Geometry check sheet. Reference: drawing and pictorial views, mm from the part's lowest x, y, z. A direction names the side the tool comes from. Give positions to 0.01 mm unless a question says otherwise; leave off trailing zeros. Write each loop counter-clockwise with the first axis right and the second up, starting at its lowest first coordinate (ties: lowest second). Pieces come first, ordered by that corner, then holes. Notation, with made-up numbers: M 14.5,-2.5 L 71.5,-2.5 A14 ccw 71.5,22.5 Z; hole C 50,51.5 d10. An arc over 180 degrees is marked long. Write item = value, one per line. Start each with the question number.
1) Cross-section at D-D, the plane x = 31. Record the cut outline in (y, z).
2) Cross-section at C-C, the plane z = 6. Record the cut outline in (x, y), plus the area to 3 significant figures.
3) Go/stop test with flat-tipped pins: pin 1 (1.5 mm diameter, centred on x = 13.5, y = 30.5, fed in from -Z); pin 2 (5 mm diameter, centred on x = 9.5, z = 20.5, fed in from +Y); pin 3 (12 mm diameter, centred on x = 8.5, y = 18.5, fed in from -Z); pin 4 (0.9 mm diameter, centred on x = 5.5, y = 36.5, fed in from -Z). Record where each tip stops, or that it passes through.
4) Access from +Z, -Z, +X, -X, +Y, -Y to the whole of each face (thin tool, end or side, straight path). Record for the marked faces 1 and 2.
5) Scan lines: line 1 along Y through (x, z) = (5.5, 24.4); line 2 along Y through (x, z) = (36, 24). Record each from-to range of solid material in increasing order. Write a range as [from, to].
6) Cross-section at A-A, the plane x = 21. Record the cut outline in (y, z).
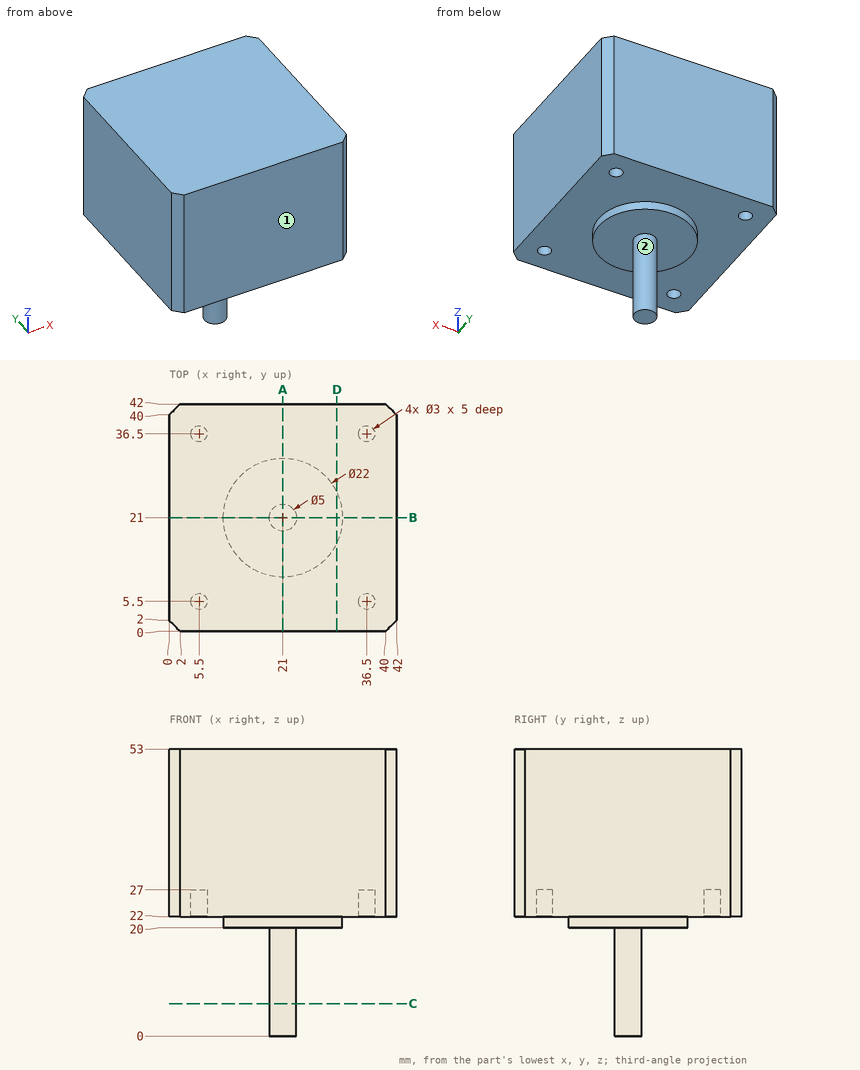
Reply:
q1.outline = M 0,22 L 16.42,22 L 16.42,20 L 25.58,20 L 25.58,22 L 42,22 L 42,53 L 0,53 Z
q2.outline = C 21,21 d5
q2.area = 19.6 mm2
q3.pin_1 = 22
q3.pin_2 = 42
q3.pin_3 = 20
q3.pin_4 = 27
q4.face_1 = +Z, -Z, +X, -X, -Y
q4.face_2 = -Z
q5.line_1 = [0, 4], [7, 35], [38, 42]
q5.line_2 = [0, 4.09], [6.91, 35.09], [37.91, 42]
q6.outline = M 0,22 L 10,22 L 10,20 L 18.5,20 L 18.5,0 L 23.5,0 L 23.5,20 L 32,20 L 32,22 L 42,22 L 42,53 L 0,53 Z
